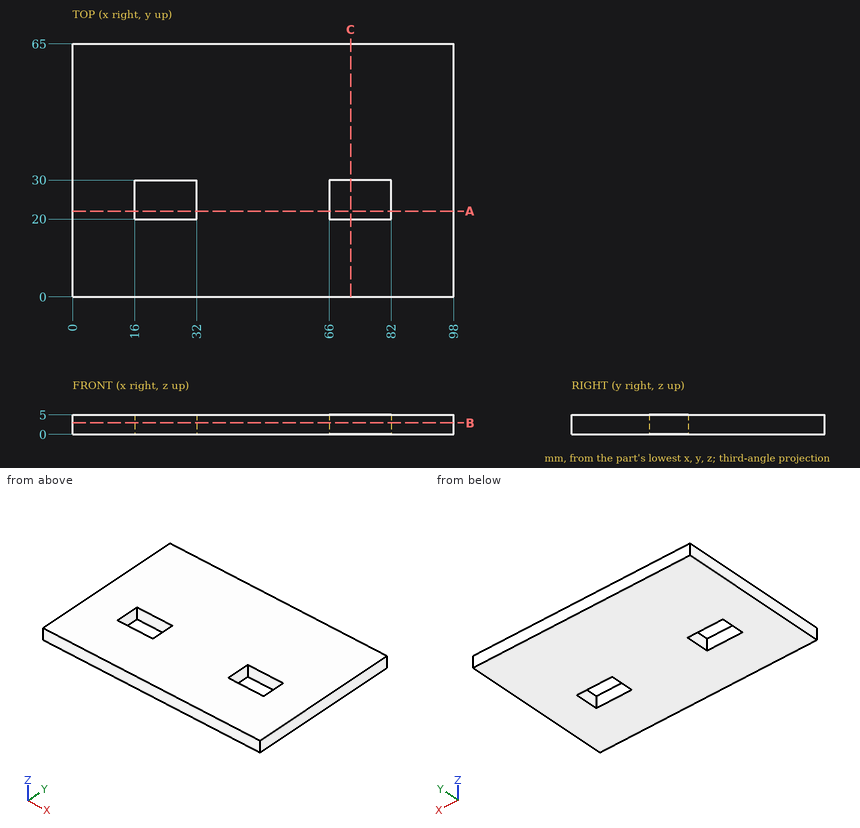
Could you check a few things on this drawing? It's one solid part, dimensions in mm from its lowest x, y, z. Give positions to 0.01 mm unless a question says otherwise; leave off trailing zeros. Write each loop counter-clockwise with the first axis right and the second up, starting at its lowest first coordinate (ties: lowest second). Pieces come first, ordered by that corner, then holes. Notation, with made-up numbers: (51, 38.5) -> (70, 38.5) arc R12 ccw to (70, 55.5) -> close; hole circle Ø6 at (89, -24.5). An arc over 180 degrees is marked (long way). Answer as CSV lines item,"result". Start each with the question number.
(1) If we section it at A-A, the plane y = 22: Write out the boundary of the cut face in (x, z).
(2) I'm going to push a flat-ended pin straight in: pin 1 Ø1.5 at (y, z) = (26.5, 2) entering from -X. Where does the tip first touch, or does it pass through?
(3) Please list where these lines run through material, in increasing order: line 1 (X direction, y = 26, z = 3.55); line 2 (Y direction, x = 22, z = 2.2).
(4) If we section it at B-B, the plane z = 2.95: Write out the boundary of the cut face in (x, y), and give its area (3 significant figures).
(5) If we section it at C-C, the plane x = 71.5: Write out the boundary of the cut face in (y, z).
Answer list:
1,outline,"(0, 0) -> (16, 0) -> (16, 5) -> (0, 5) -> close; (32, 0) -> (66, 0) -> (66, 5) -> (32, 5) -> close; (82, 0) -> (98, 0) -> (98, 5) -> (82, 5) -> close"
2,pin 1,"x = 0"
3,line 1,"0 to 16, 32 to 66, 82 to 98"
3,line 2,"0 to 20, 30 to 65"
4,outline,"(0, 0) -> (98, 0) -> (98, 65) -> (0, 65) -> close; hole (16, 20) -> (32, 20) -> (32, 30) -> (16, 30) -> close; hole (66, 20) -> (82, 20) -> (82, 30) -> (66, 30) -> close"
4,area,"6,050 mm^2"
5,outline,"(0, 0) -> (20, 0) -> (20, 5) -> (0, 5) -> close; (30, 0) -> (65, 0) -> (65, 5) -> (30, 5) -> close"
